Autodesk Inventor part; units mm, degrees
ref_plane "YZ Plane" through (0, 0, 0) normal (1, 0, 0) x (0, 1, 0)
ref_plane "XZ Plane" through (0, 0, 0) normal (0, 1, 0) x (-1, 0, 0)
ref_plane "XY Plane" through (0, 0, 0) normal (0, 0, 1) x (1, 0, 0)
sketch "スケッチ1" plane through (0, 0, 0) normal (1, 0, 0) x (0, 1, 0)
  line L0 (0, 0) -> (0, -10)
  line L1 (0, 0) -> (40, 0)
  line L2 (0, -10) -> (40, -10)
  line L3 (40, 0) -> (30, -10)
  line L4 (40, -10) -> (30, 0)
  circle A0 centre (37.8284, -5) radius 2
  line L5 (0, 0) -> (40, 0)
  line L6 (40, 0) -> (40, 1.5)
  line L7 (40, 1.5) -> (0, 1.5)
  line L8 (0, 1.5) -> (0, 0)
  line L9 (0, -10) -> (40, -10)
  line L10 (40, -10) -> (40, -11.5)
  line L11 (40, -11.5) -> (0, -11.5)
  line L12 (0, -11.5) -> (0, -10)
  point P0 (36.4142, -6.4142)
  point P1 (36.4142, -3.5858)
  dimension "d0" = 10
  dimension "d1" = 40
  dimension "d2" = 40
  dimension "d3" = 45
  dimension "d4" = 45
  dimension "d5" = 2
  dimension "d6" = 2
  dimension "d7" = 1.5
  dimension "d8" = 1.5
  dimension "d41" = 40
revolve "回転1" add sketch "スケッチ1" angle 360 about axis through (0, 0, 0) along (0, 0, -1) contours L1 L4 L3 L2 L0 | L8 L7 L6 L1 | L2 L10 L11 L12 | L1 L3 L4 | L3 L4 L2 | L3 A0 L4
sketch "スケッチ2" plane through (0, 0, 1.5) normal (0, 0, 1) x (1, 0, 0)
  point P0 (0, 0)
  point P1 (0, 0)
hole "穴1" at (0, 0, 1.5) direction (0, 0, -1) diameter 6.5 end through all
sketch "スケッチ3" plane through (0, 0, 1.5) normal (0, 0, 1) x (1, 0, 0)
  circle A0 centre (0, 0) radius 10
  line L0 (-9, 0) -> (9, 0)
  line L1 (9, 0) -> (9, -9)
  line L2 (9, -9) -> (-9, -9)
  line L3 (-9, -9) -> (-9, 0)
  point P0 (0, 0)
  point P1 (4.3589, -9)
  point P2 (9, -4.3589)
  point P3 (-9, -4.3589)
  point P4 (-4.3589, -9)
  dimension "d17" = 20
  dimension "d36" = 18
  dimension "d37" = 9
  dimension "d38" = 9
  dimension "d39" = 0
extrude "押し出し1" cut sketch "スケッチ3" against normal blind 8
sketch "スケッチ4" plane through (0, 0, 1.5) normal (0, 0, 1) x (1, 0, 0)
  point P0 (0, 0)
sketch "スケッチ5" plane through (0, 0, -11.5) normal (0, 0, -1) x (-1, 0, 0)
  circle A0 centre (0, 0) radius 6
  point P0 (0, 0)
  point P1 (6, 0)
  point P2 (0, 6)
  point P3 (-6, 0)
  point P4 (0, -6)
  dimension "d20" = 12
  dimension "d23" = 360
hole "穴2" at (-6, 0, -11.5) at (0, 6, -11.5) at (6, 0, -11.5) at (0, -6, -11.5) direction (0, 0, 1) diameter 2.5 end through all
fillet "フィレット2" radius 1 6 edges at (0, 10, 1.5) (-9, -6.6794, 1.5) (-6.6794, -9, 1.5) (0, -10, 1.5) (6.6794, -9, 1.5) (9, -6.6794, 1.5)
sketch "スケッチ7" plane through (0, 0, 1.5) normal (0, 0, 1) x (1, 0, 0)
  circle A0 centre (0, 0) radius 40
  point P0 (0, 38)
  dimension "d42" = 38
hole "穴3" at (0, 38, 1.5) direction (0, 0, -1) diameter 2.5 end through all
equation "\"d2\" = d1"
equation "\"d6\" = d5"
equation "\"d8\" = d7"
equation "\"d41\" = d1"
properties part number "s_base7"
Design review of the part built by this model. Coordinates are the model's own, in mm. A direction names the side the tool comes from. Coordinates: 2 decimals unless noted, no trailing zeros. One line per item, written item: value. Start each with the question number.
Q1. Insertion check: pin 1 Ø1.5 at (y, z) = (-22.5, -8) entering from -X; pin 2 Ø4 at (y, z) = (-24, -3) entering from -X; pin 3 Ø3.5 at (y, z) = (-6, -4) entering from -X; pin 4 Ø3 at (x, y) = (0, 38) entering from -Z. Each pin has a flat end and moves straight along its axis. Give the tip position at first contact, or say it passes through.
Q2. Take a section at A-A, the plane x = 0. Give the number of separate pieces and of enclosed holes in the cut face, then the cut area to 3 significant figures.
Q3. Tool access review of faces 1 (the conical face through (-11.005, 34.947, -3.361)), 2 (the flat face through (7, -9, -3)), 3 (the flat face through (-8, 8, 1.5)): name each direction out of +Z, -Z, +X, -X, +Y, -Y from which nothing blocks a thin tool from reaching the whole face with its end or side.
Q4. Mouldability with a two-part tool opening along X and no side actions: class faces 4 (the cylindrical face through (-0.38, 36.81, -9.69)), 5 (the flat face through (-7, -9, -3)), 6 (the conical face through (11.005, 34.947, -6.639)), 7 (the flat face through (1, 8, -11.5)) as pulls with the +X half, pulls with the -X half, needs draft (parallel to the pull), parting line crosses it, or undercut.
Q5. For probe 1 along X at (y, z) = (0, -9.9); probe 2 along Y at (x, z) = (0, -1.35); probe 3 along Y at (x, z) = (-7.5, -2), list the stretches that pass through material, from the lowest coordinate up.
Values follow:
1. pin 1: stops at x = -31.69
1. pin 2: stops at x = -31.16
1. pin 3: stops at x = -37.29
1. pin 4: stops at z = -11.5
2. separate pieces: 6
2. enclosed holes: 0
2. area: 756 mm2
3. face 1: none
3. face 2: +Z
3. face 3: +Z, +X, -X, +Y, -Y
4. face 4: undercut
4. face 5: undercut
4. face 6: parting line crosses it
4. face 7: needs draft
5. probe 1: x = -39.9 to -7.25, -4.75 to -3.25, 3.25 to 4.75, 7.25 to 39.9
5. probe 2: y = -38.65 to -10, 10 to 36.75
5. probe 3: y = -37.25 to -9, 6.61 to 37.25
